Can you work these out from the model? Positions are in its coordinate system, mm. Face numbers are marked on the shaded views. A direction names the side the tool comes from. Give positions to 0.01 mm unless a question says otherwise; leave off trailing zeros. Write each loop counter-clockwise with the first axis right and the second up, starting at its lowest first coordinate (ties: lowest second). Pieces come first, ordered by that corner, then holes. Notation, with made-up numbers: M 82,86.5 L 105,86.5 A13 cw 105,99.5 Z; hole C 53.5,38 d7. An arc over 180 degrees is marked long. Write each question's results on one line, items separated by ' | '.
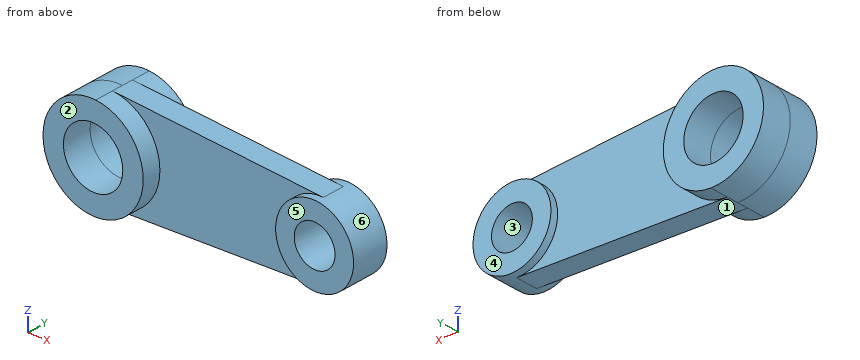
from build123d import *

# Parameters (mm, degrees)
F1_DEPTH = 9.525
F0_R     = 17.4625
F2_DEPTH = 15.875
F0_R_2   = 25.4
F3_DEPTH = 25.4


with BuildPart() as f1:
    # F0 (on Front) → F1 (new body, symmetric)
    with BuildSketch(Plane.XZ):
        with BuildLine():
            ThreePointArc((-150.9907119117, 42.803092487), (-122.150907194, 29.4999956791), (-110.3841329643, 0))
            ThreePointArc((-110.3841329643, 0), (-122.150907194, -29.4999956791), (-150.9907119117, -42.803092487))
            Line((-150.9907119117, -42.803092487), (29.4829722989, -33.2912941566))
            ThreePointArc((29.4829722989, -33.2912941566), (-5.6091329643, 0), (29.4829722989, 33.2912941566))
            Line((29.4829722989, 33.2912941566), (-150.9907119117, 42.803092487))
        make_face()
    extrude(amount=F1_DEPTH, both=True)

    # F0 (on Front) → F2 (join, symmetric)
    with BuildSketch(Plane.XZ):
        with BuildLine():
            ThreePointArc((61.0658670357, 0), (51.9139315238, 22.9444410837), (29.4829722989, 33.2912941566))
            ThreePointArc((29.4829722989, 33.2912941566), (-5.6091329643, 0), (29.4829722989, -33.2912941566))
            ThreePointArc((29.4829722989, -33.2912941566), (51.9139315238, -22.9444410837), (61.0658670357, 0))
        make_face()
        with Locations((27.7283670357, 0)):
            Circle(F0_R, mode=Mode.SUBTRACT)
    extrude(amount=F2_DEPTH, both=True)

    # F0 (on Front) → F3 (join, symmetric)
    with BuildSketch(Plane.XZ):
        with BuildLine():
            ThreePointArc((-150.9907119117, -42.803092487), (-122.150907194, -29.4999956791), (-110.3841329643, 0))
            ThreePointArc((-110.3841329643, 0), (-122.150907194, 29.4999956791), (-150.9907119117, 42.803092487))
            ThreePointArc((-150.9907119117, 42.803092487), (-196.1091329643, 0), (-150.9907119117, -42.803092487))
        make_face()
        with Locations((-153.2466329643, 0)):
            Circle(F0_R_2, mode=Mode.SUBTRACT)
    extrude(amount=F3_DEPTH, both=True)


solid = f1.part
Item 1: I want a section at B-B, the plane x = -171.5. Please give me the cut outline in (y, z).
Geometry says:
outline: M -25.4,-38.78 L 25.4,-38.78 L 25.4,-17.66 L -25.4,-17.66 Z; M -25.4,17.66 L 25.4,17.66 L 25.4,38.78 L -25.4,38.78 Z
Item 2: I want a section at A-A, the plane z = 0. Please give me the cut outline in (x, y) (3 decimals).
Geometry says:
outline: M -196.109,-25.4 L -178.647,-25.4 L -178.647,25.4 L -196.109,25.4 Z; M -127.847,-25.4 L -110.384,-25.4 L -110.384,-9.525 L -5.609,-9.525 L -5.609,-15.875 L 10.266,-15.875 L 10.266,15.875 L -5.609,15.875 L -5.609,9.525 L -110.384,9.525 L -110.384,25.4 L -127.847,25.4 Z; M 45.191,-15.875 L 61.066,-15.875 L 61.066,15.875 L 45.191,15.875 Z
Item 3: I'm going to push flat-ended pins straight in: pin 1 (2 mm diameter, centred on y = 4.5, z = 11, fed in from +X); pin 2 (1 mm diameter, centred on x = -21.5, y = 0, fed in from +Z); pin 3 (8 mm diameter, centred on y = 12, z = 30, fed in from +X). Where does each tip first touch, or does it pass through?
Geometry says:
pin 1: stops at x = 59.53 | pin 2: stops at z = 36 | pin 3: stops at x = 48.59
Item 4: For the marked faces 4, 5 and 6, which set-ups out of +Z, -Z, +X, -X, +Y, -Y let a thin tool reach every point of the face, with its end or its side?
Geometry says:
face 4: +Z, -Z, +X, +Y | face 5: +Z, -Z, +X, -Y | face 6: none
Item 5: Thinking about a two-plate mould opening in X: for the marked faces 1, 2 and 3, which applies, +X half, -X half, draft (parallel to the pull), parting line (faces both ways), or undercut?
Geometry says:
face 1: +X half | face 2: draft | face 3: undercut
Item 6: I want a section at D-D, the plane z = 30.5. Please give me the cut outline in (x, y) (3 decimals), and give its area (3 significant figures).
Geometry says:
outline: M -183.362,-25.4 L -123.131,-25.4 L -123.131,-9.525 L 14.27,-9.525 L 14.27,-15.875 L 41.187,-15.875 L 41.187,15.875 L 14.27,15.875 L 14.27,9.525 L -123.131,9.525 L -123.131,25.4 L -183.362,25.4 Z | area: 6,530 mm2
Item 7: If I drill on line 1 (X direction, y = 8.5, z = -13); line 2 (X direction, y = 1, z = -8.5); line 3 (Y direction, x = -91, z = 35) (3 decimals), over which ranges is the centre line in solid material (lowest first)? Write a range as from..to.
Geometry says:
line 1: x = -194.09..-175.07, -131.43..16.07, 39.39..58.43 | line 2: x = -195.26..-177.18, -129.31..12.47, 42.98..59.96 | line 3: y = -9.525..9.525
